from build123d import *

# Parameters (mm, degrees)
F0_R     = 6
F0_R_2   = 5
F1_DEPTH = 20
F3_DEPTH = 20
F4_R     = 6
F5_DEPTH = 5.501
F6_R     = 9.99999


# Not quite as in the source:
# - a fillet or chamfer is up to 0.001 mm smaller than in the source, because OpenCascade refuses the exact size


with BuildPart() as f1:
    # F0 (on Top) → F1 (new body)
    with BuildSketch(Plane.XY):
        Circle(F0_R)
        Circle(F0_R_2, mode=Mode.SUBTRACT)
    extrude(amount=F1_DEPTH)

    # F2 (on face) → F3 (join)
    with BuildSketch(Plane.XY.offset(20)):
        with BuildLine():
            Line((0.5, -6), (0.5, -31))
            Line((0.5, -31), (2.5, -31))
            Line((2.5, -31), (2.5, -6))
            Line((2.5, -6), (2.5, -5.4543560573))
            ThreePointArc((2.5, -5.4543560573), (1.52277609, -5.8035465863), (0.5, -5.9791303716))
            Line((0.5, -5.9791303716), (0.5, -6))
        make_face()
    extrude(amount=-F3_DEPTH)

    # F4 (on face) → F5 (cut, through all)
    with BuildSketch(Plane(origin=(0.5, 0, 0), x_dir=(0, -1, 0), z_dir=(-1, 0, 0))):
        with Locations((20.9791303716, 10)):
            Circle(F4_R)
    extrude(amount=-F5_DEPTH, mode=Mode.SUBTRACT)

    # F6 (radius 10 in the source; OpenCascade refuses exactly that, so slightly less here)
    f6_edges = [f1.edges().sort_by_distance(p)[0] for p in [
        (1.5, -31, 20),
        (1.5, -31, 0),
    ]]
    fillet(f6_edges, radius=F6_R)


solid = f1.part
CAD build for the part. Positions are in the model's coordinates, mm. A direction names the side the tool comes from. Give positions to 0.01 mm unless a question says otherwise; leave off trailing zeros. Loops run counter-clockwise (first coordinate to the right, second up) from the corner with the lowest first, then second, coordinate; pieces in that order, holes last. Notation, with made-up numbers: M -12.5,-18 L 43.5,-18 A11 cw 43.5,-2 Z; hole C 19.5,85 d1. An arc over 180 degrees is marked long. One line per question, with ' | ' between items. Start each with the question number.
1. Saw through at D-D on x = 1.75. State how many separate pieces and enclosed holes the cut face has, plus the area to 3 significant figures.
2. Probe L1, parallel to Y at x = 0, z = 12.5; L2, parallel to X at y = -12.5, z = 1.5; L3, parallel to Z at x = 1.75, y = -17. List the from-to ranges inside material, lowest first. Write a range as from..to.
3. 3-axis set-ups, long thin cutter, end or side, ignore diameter. For faces 5 (the face through (0.9, -5.4, 0)), 6 (the face through (2.5, -13, 10)): which of +Z, -Z, +X, -X, +Y, -Y reach the whole face in a straight line?
4. Saw through at A-A on y = 0. Give the cut face in (x, z), plus the area to 3 significant figures.
5. Saw through at B-B on z = 13.25. Give the cut face in (x, y).
6. Two-plate mould, pull along Z, no slides. Class faces 1 (the face through (1.51, -27.99, 2.85)), 2 (the face through (1.49, -26.52, 7.7)), 3 (the face through (1.51, -27.99, 17.15)), 4 (the face through (-1.28, 5.86, 9.86)): pulls with the +Z half, pulls with the -Z half, needs draft (parallel to the pull), parting line crosses it, or undercut.
7. Flat gauge pins, fed straight in: pin 1 (10 mm diameter, centred on y = -19, z = 8, fed in from -X); pin 2 (4 mm diameter, centred on x = -3.5, y = -8.5, fed in from +Z); pin 3 (6 mm diameter, centred on y = -26, z = 15, fed in from +X); pin 4 (1 mm diameter, centred on y = -0.5, z = 4.5, fed in from -X). Where does each tip first touch, or does it go through?
Result sheet:
1) separate pieces: 2 | enclosed holes: 1 | area: 391 mm^2
2) L1: y = -6..-5, 5..6 | L2: x = 0.5..2.5 | L3: z = 0..5.51, 14.49..20
3) face 5: -Z, +X, -X, +Y, -Y | face 6: +Z, -Z, +X, -Y
4) outline: M -6,0 L -5,0 L -5,20 L -6,20 Z; M 5,0 L 6,0 L 6,20 L 5,20 Z | area: 40.0 mm^2
5) outline: M 0.5,-30.46 L 2.5,-30.46 L 2.5,-26.02 L 0.5,-26.02 Z; M 0.5,-15.94 L 2.5,-15.94 L 2.5,-5.45 A6 ccw long 0.5,-5.98 Z; hole C 0,0 d10
6) face 1: pulls with the -Z half | face 2: undercut | face 3: pulls with the +Z half | face 4: needs draft
7) pin 1: stops at x = 0.5 | pin 2: passes through | pin 3: stops at x = 2.5 | pin 4: stops at x = -6
